CAD build for the part. Positions are in the model's coordinates, mm. Coordinates: 2 decimals unless noted, no trailing zeros. Order: outer loops, then holes, each group sorted by start corner. A loop starts at its lowest first (then second) coordinate and runs counter-clockwise, first axis right, second up. Notation, with made-up numbers: (-37.5, 88.5) - (-1.5, 88.5) arc R21 cw to (-1.5, 103.5) - close; hole circle Ø7 at (58.25, 21). An arc over 180 degrees is marked (long way). Return JSON: item names as keys, results as strings.
from build123d import *

# Parameters (mm, degrees)
SKETCH_W                          = 5.08
SKETCH_H                          = 7.62
PAD_DEPTH                         = 2.54
SKETCH001_W                       = 0.64
SKETCH001_H                       = 0.64
PAD001_DEPTH                      = 13.208
PAD001_DEPTH_BACK                 = 5.334
SKETCH001_LINEARPATTERN_2_W       = 0.64
SKETCH001_LINEARPATTERN_2_H       = 0.64
PAD001_LINEARPATTERN_2_DEPTH      = 13.208
PAD001_LINEARPATTERN_2_DEPTH_BACK = 5.334
SKETCH001_LINEARPATTERN_3_W       = 0.64
SKETCH001_LINEARPATTERN_3_H       = 0.64
PAD001_LINEARPATTERN_3_DEPTH      = 13.208
PAD001_LINEARPATTERN_3_DEPTH_BACK = 5.334
LINEARPATTERN001_COUNT            = 2
LINEARPATTERN001_PITCH            = 2.54


with BuildPart() as part:
    # Sketch → Pad (new body)
    with BuildSketch(Plane.XY):
        with Locations((1.27, -2.54)):
            Rectangle(SKETCH_W, SKETCH_H)
    extrude(amount=PAD_DEPTH)

    # Sketch001 (on Face6 of Pad) → Pad001 (join, two sides)
    with BuildSketch(Plane.XY.offset(2.54)) as pad001_sk:
        Rectangle(SKETCH001_W, SKETCH001_H)
    pad001 = extrude(amount=PAD001_DEPTH) + extrude(pad001_sk.sketch, amount=-PAD001_DEPTH_BACK)

    # Sketch001 LinearPattern 2 → Pad001 LinearPattern 2 (add, two sides)
    with BuildSketch(Plane(origin=(0, -2.54, 2.54), x_dir=(1, 0, 0), z_dir=(0, 0, 1))) as pad001_linearpattern_2_sk:
        Rectangle(SKETCH001_LINEARPATTERN_2_W, SKETCH001_LINEARPATTERN_2_H)
    pad001_linearpattern_2 = extrude(amount=PAD001_LINEARPATTERN_2_DEPTH) + extrude(pad001_linearpattern_2_sk.sketch, amount=-PAD001_LINEARPATTERN_2_DEPTH_BACK)

    # Sketch001 LinearPattern 3 → Pad001 LinearPattern 3 (add, two sides)
    with BuildSketch(Plane(origin=(0, -5.08, 2.54), x_dir=(1, 0, 0), z_dir=(0, 0, 1))) as pad001_linearpattern_3_sk:
        Rectangle(SKETCH001_LINEARPATTERN_3_W, SKETCH001_LINEARPATTERN_3_H)
    pad001_linearpattern_3 = extrude(amount=PAD001_LINEARPATTERN_3_DEPTH) + extrude(pad001_linearpattern_3_sk.sketch, amount=-PAD001_LINEARPATTERN_3_DEPTH_BACK)

    # LinearPattern001: Pad001, Pad001 LinearPattern 2, Pad001 LinearPattern 3 ×2
    with Locations(*[(i * LINEARPATTERN001_PITCH, 0, 0) for i in range(1, LINEARPATTERN001_COUNT)]):
        add(pad001)
        add(pad001_linearpattern_2)
        add(pad001_linearpattern_3)


solid = part.part
Item 1: Band-saw the part on C-C, the plane y = -6. List the corners of the cut face in (x, z), then the cut area to 3 significant figures.
Findings below:
{"outline": "(-1.27, 0) - (3.81, 0) - (3.81, 2.54) - (-1.27, 2.54) - close", "area": "12.9 mm²"}
Item 2: Drop flat-ended pins along their axis: P1, Ø0.5, axis at x = 0, z = 8, coming from the -Y side; P2, Ø0.5, axis at x = 2.5, z = 8.5, coming from the +Y side; P3, Ø3, axis at y = -3.5, z = 8, coming from the -X side. Give the stop position or say it passes through.
Findings below:
{"P1": "stops at y = -5.4", "P2": "stops at y = 0.32", "P3": "stops at x = -0.32"}
Item 3: Band-saw the part on B-B, the plane x = -0.15. List the corners of the cut face in (y, z).
Findings below:
{"outline": "(-6.35, 0) - (-5.4, 0) - (-5.4, -2.79) - (-4.76, -2.79) - (-4.76, 0) - (-2.86, 0) - (-2.86, -2.79) - (-2.22, -2.79) - (-2.22, 0) - (-0.32, 0) - (-0.32, -2.79) - (0.32, -2.79) - (0.32, 0) - (1.27, 0) - (1.27, 2.54) - (0.32, 2.54) - (0.32, 15.75) - (-0.32, 15.75) - (-0.32, 2.54) - (-2.22, 2.54) - (-2.22, 15.75) - (-2.86, 15.75) - (-2.86, 2.54) - (-4.76, 2.54) - (-4.76, 15.75) - (-5.4, 15.75) - (-5.4, 2.54) - (-6.35, 2.54) - close"}
Item 4: Wall check: L1, parallel to Y at x = 2.7, z = -1; L2, parallel to X at y = -5, z = 6.25; L3, parallel to Z at x = 1.2, y = -3.25. Give the ranges that are in metal, low to high. Write a range as [from, to].
Findings below:
{"L1": "y = [-5.4, -4.76], [-2.86, -2.22], [-0.32, 0.32]", "L2": "x = [-0.32, 0.32], [2.22, 2.86]", "L3": "z = [0, 2.54]"}
Item 5: Band-saw the part on A-A, the plane z = -0.5. List the corners of the cut face in (x, y).
Findings below:
{"outline": "(-0.32, -5.4) - (0.32, -5.4) - (0.32, -4.76) - (-0.32, -4.76) - close; (-0.32, -2.86) - (0.32, -2.86) - (0.32, -2.22) - (-0.32, -2.22) - close; (-0.32, -0.32) - (0.32, -0.32) - (0.32, 0.32) - (-0.32, 0.32) - close; (2.22, -5.4) - (2.86, -5.4) - (2.86, -4.76) - (2.22, -4.76) - close; (2.22, -2.86) - (2.86, -2.86) - (2.86, -2.22) - (2.22, -2.22) - close; (2.22, -0.32) - (2.86, -0.32) - (2.86, 0.32) - (2.22, 0.32) - close"}
